```python
from build123d import *

# Parameters (mm, degrees)
BOSS_EXTRUDE1_DEPTH = 18.25625
SKETCH2_R           = 9.5377
CUT_EXTRUDE1_DEPTH  = 59.232550302
BOSS_EXTRUDE2_START = 19.84375
BOSS_EXTRUDE2_DEPTH = 19.84375
BOSS_EXTRUDE3_DEPTH = 19.84375
FILLET2_R           = 6.35
FILLET3_R           = 3.175
FILLET5_R           = 1.5875
FILLET6_R           = 3.175


with BuildPart() as part:
    # Sketch1 → Boss-Extrude1 (new, symmetric)
    with BuildSketch(Plane.XY):
        with BuildLine():
            Line((1.403672164, 19.691144131), (4.869734215, 19.691144131))
            ThreePointArc((4.869734215, 19.691144131), (3.208035766, -4.121355869), (4.869734215, -27.933855869))
            Line((4.869734215, -27.933855869), (0.061901788, -27.933855869))
            ThreePointArc((0.061901788, -27.933855869), (-1.356220949, -12.477586426), (-1.408740732, 3.043514659))
            ThreePointArc((-1.408740732, 3.043514659), (-3.712015543, 7.317965291), (-8.567418141, 7.350655889))
            ThreePointArc((-8.567418141, 7.350655889), (-28.755262527, 25.645771293), (-1.718407463, 22.288871403))
            ThreePointArc((-1.718407463, 22.288871403), (-0.627064659, 20.425502216), (1.403672164, 19.691144131))
        make_face()
    extrude(amount=BOSS_EXTRUDE1_DEPTH, both=True)

    # Sketch2 → Cut-Extrude1 (cut, through all)
    with BuildSketch(Plane.XY.offset(18.25625)):
        with Locations((-15.767765785, 19.691144131)):
            Circle(SKETCH2_R)
    extrude(amount=-CUT_EXTRUDE1_DEPTH, mode=Mode.SUBTRACT)

    # Sketch4 → Boss-Extrude2 (add)
    with BuildSketch(Plane.XY.offset(18.25625).offset(BOSS_EXTRUDE2_START)):
        with BuildLine():
            ThreePointArc((-1.408740732, 3.043514659), (-1.356220949, -12.477586426), (0.061901788, -27.933855869))
            Line((0.061901788, -27.933855869), (4.869734215, -27.933855869))
            ThreePointArc((4.869734215, -27.933855869), (3.208035766, -4.121355869), (4.869734215, 19.691144131))
            Line((4.869734215, 19.691144131), (1.403672164, 19.691144131))
            ThreePointArc((1.403672164, 19.691144131), (0.737132208, 19.761897123), (0.100299146, 19.971002722))
            ThreePointArc((0.100299146, 19.971002722), (-0.858408657, 11.525461487), (-1.408740732, 3.043514659))
        make_face()
    extrude(amount=-BOSS_EXTRUDE2_DEPTH)

    # Sketch5 → Boss-Extrude3 (add)
    with BuildSketch(Plane(origin=(0, 0, -18.25625), x_dir=(-1, 0, 0), z_dir=(0, 0, -1))):
        with BuildLine():
            ThreePointArc((-4.869734215, 19.691144131), (-3.208035766, -4.121355869), (-4.869734215, -27.933855869))
            Line((-4.869734215, -27.933855869), (-0.061901788, -27.933855869))
            ThreePointArc((-0.061901788, -27.933855869), (1.356220949, -12.477586426), (1.408740732, 3.043514659))
            ThreePointArc((1.408740732, 3.043514659), (0.858408657, 11.525461487), (-0.100299146, 19.971002722))
            ThreePointArc((-0.100299146, 19.971002722), (-0.737132208, 19.761897123), (-1.403672164, 19.691144131))
            Line((-1.403672164, 19.691144131), (-4.869734215, 19.691144131))
        make_face()
    extrude(amount=BOSS_EXTRUDE3_DEPTH)

    # Fillet2
    fillet2_edges = [part.edges().sort_by_distance(p)[0] for p in [
        (2.465818001, -27.933855869, 38.1),
        (2.465818001, -27.933855869, -38.1),
    ]]
    fillet(fillet2_edges, radius=FILLET2_R)

    # Fillet3
    # the kernel refuses this fillet: 3.175 mm, written as the material it takes off along each edge
    with BuildSketch(Plane(origin=(0.061901788, -27.933855869, 38.798080837), x_dir=(1, 0, 0), z_dir=(0, 0, -1))) as fillet3_piece_1:
        with BuildLine():
            CenterArc((2.793718395, -3.175), FILLET3_R, 90, 83.150253564)
            ThreePointArc((-0.358619505, -2.796330275), (-0.18490217, -1.39744793), (0, 0))
            Line((0, 0), (2.793718395, 0))
        make_face()
    extrude(amount=77.596161674, mode=Mode.SUBTRACT)

    # Fillet5
    # the kernel refuses this fillet: 1.5875 mm, written as the material it takes off along each edge
    with BuildSketch(Plane(origin=(0.100299146, 19.971002722, 42.300034066), x_dir=(-0.13199952505411708, -0.9912497795134622, 0), z_dir=(0, 0, -1)), Plane(origin=(0.100299146, 19.971002722, -18.25625), x_dir=(-0.1319995250540647, -0.9912497795134693, 0), z_dir=(0, 0, -1))) as fillet5_piece_1:
        with BuildLine():
            CenterArc((1.672445997, -1.587481962), FILLET5_R, 89.726869391, 82.687978074)
            Line((0.098836972, -1.377932716), (-0.05852393, -1.356977792))
            ThreePointArc((-0.05852393, -1.356977792), (-0.051995755, -1.307954493), (-0.152092645, -0.045490546))
            Line((-0.152092645, -0.045490546), (-0.000756763, 0.158748196))
            ThreePointArc((-0.000756763, 0.158748196), (0.840006813, 0.160752172), (1.680770389, 0.158748196))
            Line((1.680770389, 0.158748196), (1.680013626, 0))
        make_face()
    extrude(amount=24.043784066, mode=Mode.SUBTRACT)

    # Fillet6
    # the kernel refuses this fillet: 3.175 mm, written as the material it takes off along each edge
    with BuildSketch(Plane(origin=(12.807234215, 19.691144131, 38.1), x_dir=(0, -1, 0), z_dir=(-1, 0, 0)), Plane(origin=(-6.484371786, 19.691144131, -38.1), x_dir=(0, -1, 0), z_dir=(1, 0, 0))) as fillet6_piece_1:
        with BuildLine():
            CenterArc((FILLET6_R, -FILLET6_R), FILLET6_R, 90, 90)
            Line((0, -FILLET6_R), (0, 0))
            Line((0, 0), (FILLET6_R, 0))
        make_face()
    extrude(amount=19.291606, mode=Mode.SUBTRACT)


solid = part.part
```
Work out the finished part from the listing and answer in its coordinate system (mm). A direction names the side the tool comes from. Give positions to 0.01 mm unless a question says otherwise; leave off trailing zeros. Loops run counter-clockwise (first coordinate to the right, second up) from the corner with the lowest first, then second, coordinate; pieces in that order, holes last. Notation, with made-up numbers: M 41.25,55.5 L 75.25,55.5 A27 cw 75.25,90.5 Z; hole C 78.5,-17 d11. An arc over 180 degrees is marked long. One line per item, written item: value. Start each with the question number.
1. Each of these flat-tipped pins is pushed along its axis until it touches: P1, Ø17, axis at x = -15.77, y = 19.69, coming from the +Z side; P2, Ø1, axis at y = 2.5, z = -2.5, coming from the +X side; P3, Ø8, axis at x = -22, y = 27.5, coming from the +Z side; P4, Ø1, axis at x = 0, z = -16, coming from the +Y side. Where does it stop, or does it pass through?
2. Find section A-A (y = 15.5). Give the vertices of the cut face in (x, z), and give its area (3 significant figures).
3. Find section B-B (x = -20). Give the vertices of the cut face in (y, z).
4. Find the intervals of material crossed by probe 1 along Y at (x, z) = (-16, 11.5); probe 2 along X at (y, z) = (-5, -24); probe 3 along X at (y, z) = (7.5, 9.5), in increasing order.
5. Which of the six approach directions +Z, -Z, +X, -X, +Y, -Y give full straight-line access (tool end or side, diameter ignored) to faces 1 (the face through (0.39, 19.28, 28.04)), 2 (the face through (0.39, 19.28, -27.77)), 3 (the face through (3, 19.691, 0)), 4 (the face through (2.67, -26.123, -36.19))?
6. Determine the mould class of faces 5 (the face through (2.3, 18.74, 37.19)), 6 (the face through (3.21, -3.79, 0.53)), 7 (the face through (2.13, -26.024, 36.289)) for opening direction Y: released by +Y, released by -Y, zero draft, split by the parting line, or undercut.
Reported:
1. P1: passes through
1. P2: stops at x = 3.36
1. P3: stops at z = 18.26
1. P4: stops at y = 20.33
2. outline: M -29.43,-18.26 L -24.34,-18.26 L -24.34,18.26 L -29.43,18.26 Z; M -7.2,-18.26 L -0.46,-18.26 L -0.46,-38.1 L 4.33,-38.1 L 4.33,38.1 L -0.46,38.1 L -0.46,18.26 L -7.2,18.26 Z
2. area: 797 mm²
3. outline: M 6.04,-18.26 L 11.14,-18.26 L 11.14,18.26 L 6.04,18.26 Z; M 28.24,-18.26 L 33.34,-18.26 L 33.34,18.26 L 28.24,18.26 Z
4. probe 1: y = 5.41 to 10.16, 29.23 to 33.98
4. probe 2: x = -1.55 to 3.21
4. probe 3: x = -23.22 to -8.29, -4.04 to 3.6
5. face 1: +Z, -X, +Y
5. face 2: -Z, -X, +Y
5. face 3: +Z, -Z, +X, +Y
5. face 4: -Z, +X, -X, -Y
6. face 5: released by +Y
6. face 6: undercut
6. face 7: released by -Y
